from build123d import *

# Parameters (mm, degrees)
SKETCH1_W           = 45
SKETCH1_H           = 24
BOSS_EXTRUDE1_DEPTH = 18
SKETCH2_W           = 10
SKETCH2_H           = 24
CUT_EXTRUDE1_DEPTH  = 10
SKETCH3_R           = 1.6
CUT_EXTRUDE2_DEPTH  = 9
SKETCH4_R           = 3.1
CUT_EXTRUDE3_DEPTH  = 2.5
SKETCH5_W           = 14.23
SKETCH5_H           = 19
CUT_EXTRUDE4_DEPTH  = 15.5
SKETCH6_R           = 7.115
CUT_EXTRUDE5_DEPTH  = 3.5
CHAMFER1_SIZE       = 2.5


with BuildPart() as part:
    # Sketch1 → Boss-Extrude1 (new body)
    with BuildSketch(Plane(origin=(0, 0, 0), x_dir=(1, 0, 0), z_dir=(0, 1, 0))):
        Rectangle(SKETCH1_W, SKETCH1_H)
    extrude(amount=BOSS_EXTRUDE1_DEPTH)

    # Sketch2 → Cut-Extrude1 (cut)
    with BuildSketch(Plane(origin=(0, 18, 0), x_dir=(1, 0, 0), z_dir=(0, 1, 0))):
        with Locations((-17.5, 0)):
            Rectangle(SKETCH2_W, SKETCH2_H)
        with Locations((17.5, 0)):
            Rectangle(SKETCH2_W, SKETCH2_H)
    extrude(amount=-CUT_EXTRUDE1_DEPTH, mode=Mode.SUBTRACT)

    # Sketch3 → Cut-Extrude2 (cut, through all)
    with BuildSketch(Plane(origin=(0, 8, 0), x_dir=(1, 0, 0), z_dir=(0, 1, 0))):
        with Locations((-17.5, 0)):
            Circle(SKETCH3_R)
        with Locations((17.5, 0)):
            Circle(SKETCH3_R)
    extrude(amount=-CUT_EXTRUDE2_DEPTH, mode=Mode.SUBTRACT)

    # Sketch4 → Cut-Extrude3 (cut)
    with BuildSketch(Plane(origin=(0, 8, 0), x_dir=(1, 0, 0), z_dir=(0, 1, 0))):
        with Locations((-17.5, 0)):
            Circle(SKETCH4_R)
        with Locations((17.5, 0)):
            Circle(SKETCH4_R)
    extrude(amount=-CUT_EXTRUDE3_DEPTH, mode=Mode.SUBTRACT)

    # Sketch5 → Cut-Extrude4 (cut)
    with BuildSketch(Plane.XZ):
        Rectangle(SKETCH5_W, SKETCH5_H)
    extrude(amount=-CUT_EXTRUDE4_DEPTH, mode=Mode.SUBTRACT)

    # Sketch6 → Cut-Extrude5 (cut, through all)
    with BuildSketch(Plane.XZ.offset(-15.5)):
        with Locations((0, -2.385)):
            Circle(SKETCH6_R)
    extrude(amount=-CUT_EXTRUDE5_DEPTH, mode=Mode.SUBTRACT)

    # Chamfer1
    chamfer1_edges = [part.edges().sort_by_distance(p)[0] for p in [
        (-22.5, 4, -12),
        (22.5, 4, -12),
        (22.5, 4, 12),
        (-22.5, 4, 12),
        (-12.5, 13, 12),
        (-12.5, 13, -12),
        (12.5, 13, -12),
        (12.5, 13, 12),
    ]]
    chamfer(chamfer1_edges, length=CHAMFER1_SIZE)


solid = part.part
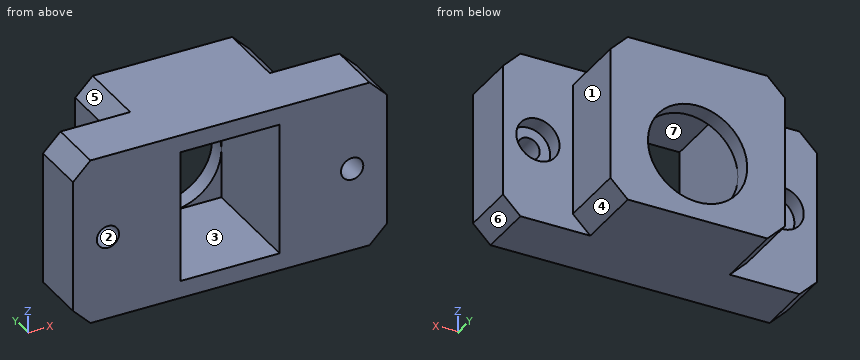
The model under review builds one solid part; all positions refer to its coordinate system, in mm. Face numbers are marked on the shaded views. A direction names the side the tool comes from. Coordinates: 2 decimals unless noted, no trailing zeros. Order: outer loops, then holes, each group sorted by start corner. A loop starts at its lowest first (then second) coordinate and runs counter-clockwise, first axis right, second up. Notation, with made-up numbers: (-32.5, -7.75) -> (-28.5, -7.75) arc R29 ccw to (-28.5, 16.25) -> close; hole circle Ø10 at (13, 45). An arc over 180 degrees is marked (long way). Answer in a Markdown table with one row per item.
(1) Consider section C-C (z = -7.75). Write out the cut boundary in (x, y) (3 decimals).
Answers:
| item | result |
|---|---|
| outline | (-22.5, 0) -> (-7.115, 0) -> (-7.115, 15.5) -> (-4.673, 15.5) -> (-4.673, 18) -> (-12.5, 18) -> (-12.5, 8) -> (-22.5, 8) -> close; (4.673, 15.5) -> (7.115, 15.5) -> (7.115, 0) -> (22.5, 0) -> (22.5, 8) -> (12.5, 8) -> (12.5, 18) -> (4.673, 18) -> close |
(2) Consider section A-A (y = 6). Write out the cut boundary in (x, z) (3 decimals).
Answers:
| item | result |
|---|---|
| outline | (-22.5, -9.5) -> (-20, -12) -> (20, -12) -> (22.5, -9.5) -> (22.5, 9.5) -> (20, 12) -> (-20, 12) -> (-22.5, 9.5) -> close; hole circle Ø6.2 at (-17.5, 0); hole (-7.115, -9.5) -> (7.115, -9.5) -> (7.115, 9.5) -> (-7.115, 9.5) -> close; hole circle Ø6.2 at (17.5, 0) |
(3) Wall thickness on line 1 along X through (y, z) = (7, -0.25) (3 decimals); line 2 along Z through (x, y) = (17.5, 2); line 3 along X through (y, z) = (13.5, 9.25) (3 decimals): over which ranges is each line inside the solid? List them lowest first.
Answers:
| item | result |
|---|---|
| line 1 | -22.5 to -20.59, -14.41 to -7.115, 7.115 to 14.41, 20.59 to 22.5 |
| line 2 | -12 to -1.6, 1.6 to 12 |
| line 3 | -12.5 to -7.115, 7.115 to 12.5 |
(4) Consider section B-B (x = 17.5). Write out the cut boundary in (y, z).
Answers:
| item | result |
|---|---|
| outline | (0, -12) -> (8, -12) -> (8, -3.1) -> (5.5, -3.1) -> (5.5, -1.6) -> (0, -1.6) -> close; (0, 1.6) -> (5.5, 1.6) -> (5.5, 3.1) -> (8, 3.1) -> (8, 12) -> (0, 12) -> close |
(5) Machinability: for the marked faces 1, 2, 3 and 4, which of the approach directions +Z, -Z, +X, -X, +Y, -Y give a long, thin tool a straight path to every point of the face, cutting with its end or side? Answer none if there is none.
Answers:
| item | result |
|---|---|
| face 1 | +Z, -Z, +X, +Y |
| face 2 | +Y, -Y |
| face 3 | -Y |
| face 4 | -Z, +X, +Y |
(6) The part is to be moulded in two halves that separate along X. For the marked faces 5, 6 and 7, say which applies: +X half, -X half, draft (parallel to the pull), parting line (faces both ways), or undercut.
Answers:
| item | result |
|---|---|
| face 5 | -X half |
| face 6 | +X half |
| face 7 | undercut |
(7) Insertion check: pin 1 (7 mm diameter, centred on x = 18.5, z = 0, fed in from +Y); pin 2 (3 mm diameter, centred on x = 17.5, z = 0, fed in from +Y); pin 3 (4 mm diameter, centred on x = -17.5, z = 0, fed in from +Y); pin 4 (5 mm diameter, centred on x = 14, y = 13.5, fed in from -Z). Each pin has a flat end and moves straight along its axis. Give the tip position at first contact, or say it passes through.
Answers:
| item | result |
|---|---|
| pin 1 | y = 8 |
| pin 2 | through |
| pin 3 | y = 5.5 |
| pin 4 | z = -10.5 |
(8) Consider section D-D (y = 12.25). Write out the cut boundary in (x, z) (3 decimals).
Answers:
| item | result |
|---|---|
| outline | (-12.5, -9.5) -> (-10, -12) -> (10, -12) -> (12.5, -9.5) -> (12.5, 9.5) -> (10, 12) -> (-10, 12) -> (-12.5, 9.5) -> close; hole (-7.115, -9.5) -> (7.115, -9.5) -> (7.115, 9.5) -> (-7.115, 9.5) -> close |
